Design review of the part built by this model. Coordinates are the model's own, in mm. A direction names the side the tool comes from. Round coordinates to 2 decimals unless told otherwise and drop trailing zeros. Use a Markdown table: item, result. Add a question column.
(1) Machinability: for faces 1 (the face through (12.7, 0, 322)), 2 (the face through (0, -9.525, 322)), which of the approach directions +Z, -Z, +X, -X, +Y, -Y give a long, thin tool a straight path to every point of the face, cutting with its end or side? Answer none if there is none.
(2) To check wall thickness, follow probe 1 along Y at (x, z) = (11.4, 247.85); probe 2 along X at (y, z) = (-11.8, 146.35); probe 3 along Y at (x, z) = (6.5, 219). State the ranges of each line that lie inside material, in increasing order. Write a range as from..to.
(3) For pin 1 (4.5 mm diameter, centred on x = -2.38, z = 552.35, fed in from +Y) (3 decimals); pin 2 (4 mm diameter, centred on y = 2.38, z = 494.35, fed in from -X) (3 decimals), all flat-tipped, find the tip position at first contact; note any pin that passes through.
(4) The part is to be moulded in two halves that separate along Z. For faces 3 (the face through (7.6, -9.5, 25.6)), 4 (the face through (6, -10, 609.6)), 5 (the face through (9.525, 1, 322)), say which applies: released by +Z, released by -Z, zero draft, split by the parting line, or undercut.
```python
from build123d import *

# Parameters (mm, degrees)
BOSS_EXTRUDE1_DEPTH = 609.6
SKETCH3_W           = 635.2
SKETCH3_H           = 25.4
CUT_EXTRUDE2_DEPTH  = 30.48
SKETCH4_R           = 1.7
CUT_EXTRUDE4_DEPTH  = 611.137198198
SKETCH7_R           = 1.7
CUT_EXTRUDE6_DEPTH  = 611.137198198
CUT_EXTRUDE7_DEPTH  = 611.137198198
CUT_EXTRUDE8_DEPTH  = 611.137198198


with BuildPart() as part:
    # Sketch2 → Boss-Extrude1 (new, symmetric)
    with BuildSketch(Plane.XY):
        with BuildLine():
            Line((-12.7, -12.7), (12.7, -12.7))
            Line((12.7, -12.7), (12.7, 12.7))
            Line((12.7, 12.7), (11.1125, 12.7))
            ThreePointArc((11.1125, 12.7), (9.989967985, 12.235032015), (9.525, 11.1125))
            Line((9.525, 11.1125), (9.525, -6.35))
            ThreePointArc((9.525, -6.35), (8.59506403, -8.59506403), (6.35, -9.525))
            Line((6.35, -9.525), (-11.1125, -9.525))
            ThreePointArc((-11.1125, -9.525), (-12.235032015, -9.989967985), (-12.7, -11.1125))
            Line((-12.7, -11.1125), (-12.7, -12.7))
        make_face()
    extrude(amount=BOSS_EXTRUDE1_DEPTH, both=True)

    # Sketch3 → Cut-Extrude2 (cut)
    with BuildSketch(Plane(origin=(12.7, 0, 0), x_dir=(0, 0, -1), z_dir=(1, 0, 0))):
        with Locations((292, 0)):
            Rectangle(SKETCH3_W, SKETCH3_H)
    extrude(amount=-CUT_EXTRUDE2_DEPTH, mode=Mode.SUBTRACT)

    # Sketch4 → Cut-Extrude4 (cut, through all)
    with BuildSketch(Plane(origin=(0, -9.525, 0), x_dir=(1, 0, 0), z_dir=(0, 1, 0))):
        with Locations(Location((-2.38125, -552.35, 0), (0, 0, 180))):
            Circle(SKETCH4_R)
        with Locations(Location((-2.38125, -537.85, 0), (0, 0, 180))):
            Circle(SKETCH4_R)
        with Locations(Location((-2.38125, -523.35, 0), (0, 0, 180))):
            Circle(SKETCH4_R)
        with Locations(Location((-2.38125, -508.85, 0), (0, 0, 180))):
            Circle(SKETCH4_R)
        with Locations(Location((-2.38125, -494.35, 0), (0, 0, 180))):
            Circle(SKETCH4_R)
        with Locations(Location((-2.38125, -479.85, 0), (0, 0, 180))):
            Circle(SKETCH4_R)
        with Locations(Location((-2.38125, -465.35, 0), (0, 0, 180))):
            Circle(SKETCH4_R)
        with Locations(Location((-2.38125, -450.85, 0), (0, 0, 180))):
            Circle(SKETCH4_R)
        with Locations(Location((-2.38125, -436.35, 0), (0, 0, 180))):
            Circle(SKETCH4_R)
        with Locations(Location((-2.38125, -421.85, 0), (0, 0, 180))):
            Circle(SKETCH4_R)
        with Locations(Location((-2.38125, -407.35, 0), (0, 0, 180))):
            Circle(SKETCH4_R)
        with Locations(Location((-2.38125, -392.85, 0), (0, 0, 180))):
            Circle(SKETCH4_R)
        with Locations(Location((-2.38125, -378.35, 0), (0, 0, 180))):
            Circle(SKETCH4_R)
        with Locations(Location((-2.38125, -363.85, 0), (0, 0, 180))):
            Circle(SKETCH4_R)
        with Locations(Location((-2.38125, -349.35, 0), (0, 0, 180))):
            Circle(SKETCH4_R)
        with Locations(Location((-2.38125, -334.85, 0), (0, 0, 180))):
            Circle(SKETCH4_R)
        with Locations(Location((-2.38125, -320.35, 0), (0, 0, 180))):
            Circle(SKETCH4_R)
        with Locations(Location((-2.38125, -305.85, 0), (0, 0, 180))):
            Circle(SKETCH4_R)
        with Locations(Location((-2.38125, -291.35, 0), (0, 0, 180))):
            Circle(SKETCH4_R)
        with Locations(Location((-2.38125, -276.85, 0), (0, 0, 180))):
            Circle(SKETCH4_R)
        with Locations(Location((-2.38125, -262.35, 0), (0, 0, 180))):
            Circle(SKETCH4_R)
        with Locations(Location((-2.38125, -247.85, 0), (0, 0, 180))):
            Circle(SKETCH4_R)
        with Locations(Location((-2.38125, -233.35, 0), (0, 0, 180))):
            Circle(SKETCH4_R)
        with Locations(Location((-2.38125, -218.85, 0), (0, 0, 180))):
            Circle(SKETCH4_R)
        with Locations(Location((-2.38125, -204.35, 0), (0, 0, 180))):
            Circle(SKETCH4_R)
        with Locations(Location((-2.38125, -189.85, 0), (0, 0, 180))):
            Circle(SKETCH4_R)
        with Locations(Location((-2.38125, -175.35, 0), (0, 0, 180))):
            Circle(SKETCH4_R)
        with Locations(Location((-2.38125, -160.85, 0), (0, 0, 180))):
            Circle(SKETCH4_R)
        with Locations(Location((-2.38125, -146.35, 0), (0, 0, 180))):
            Circle(SKETCH4_R)
        with Locations(Location((-2.38125, -131.85, 0), (0, 0, 180))):
            Circle(SKETCH4_R)
        with Locations(Location((-2.38125, -117.35, 0), (0, 0, 180))):
            Circle(SKETCH4_R)
        with Locations(Location((-2.38125, -102.85, 0), (0, 0, 180))):
            Circle(SKETCH4_R)
    extrude(amount=-CUT_EXTRUDE4_DEPTH, mode=Mode.SUBTRACT)

    # Sketch7 → Cut-Extrude6 (cut, through all)
    with BuildSketch(Plane.ZY.offset(-9.525)):
        with Locations(Location((552.35, 2.38125, 0), (0, 0, 270))):
            Circle(SKETCH7_R)
        with Locations(Location((537.85, 2.38125, 0), (0, 0, 270))):
            Circle(SKETCH7_R)
        with Locations(Location((523.35, 2.38125, 0), (0, 0, 270))):
            Circle(SKETCH7_R)
        with Locations(Location((508.85, 2.38125, 0), (0, 0, 270))):
            Circle(SKETCH7_R)
        with Locations(Location((494.35, 2.38125, 0), (0, 0, 270))):
            Circle(SKETCH7_R)
        with Locations(Location((479.85, 2.38125, 0), (0, 0, 270))):
            Circle(SKETCH7_R)
        with Locations(Location((465.35, 2.38125, 0), (0, 0, 270))):
            Circle(SKETCH7_R)
        with Locations(Location((450.85, 2.38125, 0), (0, 0, 270))):
            Circle(SKETCH7_R)
        with Locations(Location((436.35, 2.38125, 0), (0, 0, 270))):
            Circle(SKETCH7_R)
        with Locations(Location((421.85, 2.38125, 0), (0, 0, 270))):
            Circle(SKETCH7_R)
        with Locations(Location((407.35, 2.38125, 0), (0, 0, 270))):
            Circle(SKETCH7_R)
        with Locations(Location((392.85, 2.38125, 0), (0, 0, 270))):
            Circle(SKETCH7_R)
        with Locations(Location((378.35, 2.38125, 0), (0, 0, 270))):
            Circle(SKETCH7_R)
        with Locations(Location((363.85, 2.38125, 0), (0, 0, 270))):
            Circle(SKETCH7_R)
        with Locations(Location((349.35, 2.38125, 0), (0, 0, 270))):
            Circle(SKETCH7_R)
        with Locations(Location((334.85, 2.38125, 0), (0, 0, 270))):
            Circle(SKETCH7_R)
        with Locations(Location((320.35, 2.38125, 0), (0, 0, 270))):
            Circle(SKETCH7_R)
        with Locations(Location((305.85, 2.38125, 0), (0, 0, 270))):
            Circle(SKETCH7_R)
        with Locations(Location((291.35, 2.38125, 0), (0, 0, 270))):
            Circle(SKETCH7_R)
        with Locations(Location((276.85, 2.38125, 0), (0, 0, 270))):
            Circle(SKETCH7_R)
        with Locations(Location((262.35, 2.38125, 0), (0, 0, 270))):
            Circle(SKETCH7_R)
        with Locations(Location((247.85, 2.38125, 0), (0, 0, 270))):
            Circle(SKETCH7_R)
        with Locations(Location((233.35, 2.38125, 0), (0, 0, 270))):
            Circle(SKETCH7_R)
        with Locations(Location((218.85, 2.38125, 0), (0, 0, 270))):
            Circle(SKETCH7_R)
        with Locations(Location((204.35, 2.38125, 0), (0, 0, 270))):
            Circle(SKETCH7_R)
        with Locations(Location((189.85, 2.38125, 0), (0, 0, 270))):
            Circle(SKETCH7_R)
        with Locations(Location((175.35, 2.38125, 0), (0, 0, 270))):
            Circle(SKETCH7_R)
        with Locations(Location((160.85, 2.38125, 0), (0, 0, 270))):
            Circle(SKETCH7_R)
        with Locations(Location((146.35, 2.38125, 0), (0, 0, 270))):
            Circle(SKETCH7_R)
        with Locations(Location((131.85, 2.38125, 0), (0, 0, 270))):
            Circle(SKETCH7_R)
        with Locations(Location((117.35, 2.38125, 0), (0, 0, 270))):
            Circle(SKETCH7_R)
        with Locations(Location((102.85, 2.38125, 0), (0, 0, 270))):
            Circle(SKETCH7_R)
    extrude(amount=-CUT_EXTRUDE6_DEPTH, mode=Mode.SUBTRACT)

    # Sketch8 → Cut-Extrude7 (cut, through all)
    with BuildSketch(Plane.ZY.offset(-9.525)):
        with BuildLine():
            Line((49.3305, 4.0825), (52.7305, 4.0825))
            ThreePointArc((52.7305, 4.0825), (54.4305, 2.3825), (52.7305, 0.6825))
            Line((52.7305, 0.6825), (49.3305, 0.6825))
            ThreePointArc((49.3305, 0.6825), (47.6305, 2.3825), (49.3305, 4.0825))
        make_face()
        with BuildLine():
            Line((78.0325, 4.0825), (81.4325, 4.0825))
            ThreePointArc((81.4325, 4.0825), (83.1325, 2.3825), (81.4325, 0.6825))
            Line((81.4325, 0.6825), (78.0325, 0.6825))
            ThreePointArc((78.0325, 0.6825), (76.3325, 2.3825), (78.0325, 4.0825))
        make_face()
        with BuildLine():
            Line((573.7675, 4.0825), (577.1675, 4.0825))
            ThreePointArc((577.1675, 4.0825), (578.8675, 2.3825), (577.1675, 0.6825))
            Line((577.1675, 0.6825), (573.7675, 0.6825))
            ThreePointArc((573.7675, 0.6825), (572.0675, 2.3825), (573.7675, 4.0825))
        make_face()
        with BuildLine():
            Line((602.4695, 4.0825), (605.8695, 4.0825))
            ThreePointArc((605.8695, 4.0825), (607.5695, 2.3825), (605.8695, 0.6825))
            Line((605.8695, 0.6825), (602.4695, 0.6825))
            ThreePointArc((602.4695, 0.6825), (600.7695, 2.3825), (602.4695, 4.0825))
        make_face()
    extrude(amount=-CUT_EXTRUDE7_DEPTH, mode=Mode.SUBTRACT)

    # Sketch9 → Cut-Extrude8 (cut, through all)
    with BuildSketch(Plane(origin=(0, -9.525, 0), x_dir=(1, 0, 0), z_dir=(0, 1, 0))):
        with BuildLine():
            Line((-4.0825, -605.8695), (-4.0825, -602.4695))
            ThreePointArc((-4.0825, -602.4695), (-2.3825, -600.7695), (-0.6825, -602.4695))
            Line((-0.6825, -602.4695), (-0.6825, -605.8695))
            ThreePointArc((-0.6825, -605.8695), (-2.3825, -607.5695), (-4.0825, -605.8695))
        make_face()
        with BuildLine():
            Line((-4.0825, -577.1675), (-4.0825, -573.7675))
            ThreePointArc((-4.0825, -573.7675), (-2.3825, -572.0675), (-0.6825, -573.7675))
            Line((-0.6825, -573.7675), (-0.6825, -577.1675))
            ThreePointArc((-0.6825, -577.1675), (-2.3825, -578.8675), (-4.0825, -577.1675))
        make_face()
        with BuildLine():
            Line((-4.0825, -81.4325), (-4.0825, -78.0325))
            ThreePointArc((-4.0825, -78.0325), (-2.3825, -76.3325), (-0.6825, -78.0325))
            Line((-0.6825, -78.0325), (-0.6825, -81.4325))
            ThreePointArc((-0.6825, -81.4325), (-2.3825, -83.1325), (-4.0825, -81.4325))
        make_face()
        with BuildLine():
            Line((-4.0825, -52.7305), (-4.0825, -49.3305))
            ThreePointArc((-4.0825, -49.3305), (-2.3825, -47.6305), (-0.6825, -49.3305))
            Line((-0.6825, -49.3305), (-0.6825, -52.7305))
            ThreePointArc((-0.6825, -52.7305), (-2.3825, -54.4305), (-4.0825, -52.7305))
        make_face()
    extrude(amount=-CUT_EXTRUDE8_DEPTH, mode=Mode.SUBTRACT)


solid = part.part
```
Verdict:
| question | item | result |
|---|---|---|
| 1 | face 1 | +Z, -Z, +X, +Y, -Y |
| 1 | face 2 | +Z, -Z, -X, +Y |
| 2 | probe 1 | y = -12.7..0.68, 4.08..12.7 |
| 2 | probe 2 | x = -12.7..-4.08, -0.68..12.7 |
| 2 | probe 3 | y = -12.7..-9.52 |
| 3 | pin 1 | stops at y = -9.525 |
| 3 | pin 2 | stops at x = 9.525 |
| 4 | face 3 | released by -Z |
| 4 | face 4 | released by +Z |
| 4 | face 5 | zero draft |
